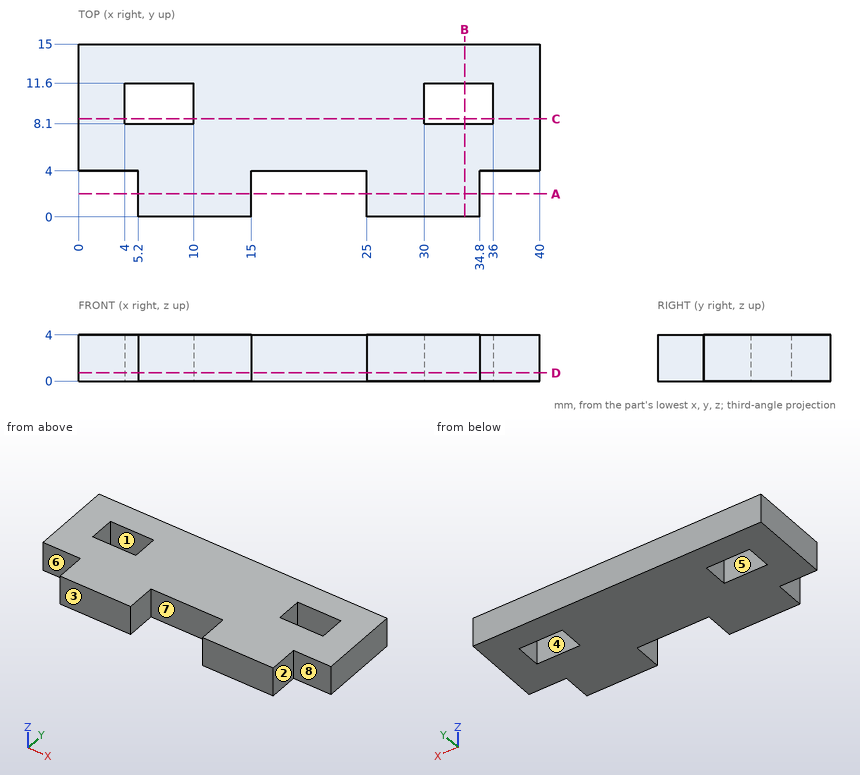
Geometry check sheet. Reference: drawing and pictorial views, mm from the part's lowest x, y, z. A direction names the side the tool comes from. Round coordinates to 2 decimals unless told otherwise and drop trailing zeros. Loops run counter-clockwise (first coordinate to the right, second up) from the corner with the lowest first, then second, coordinate; pieces in that order, holes last.
1. Sectioned sample at A-A on y = 2. Record the boundary of the cut face in (x, z).
2. Set-up check for the marked faces 5, 6, 7 and 8: record each of +Z, -Z, +X, -X, +Y, -Y from which the full face is reachable in a straight line by a thin tool's end or side.
3. Scan lines: probe 1 along X at (y, z) = (10.5, 0.2); probe 2 along Y at (x, z) = (5.5, 3.35); probe 3 along Y at (x, z) = (4.5, 3.65). Record each from-to range of solid material in increasing order.
4. Sectioned sample at C-C on y = 8.5. Record the boundary of the cut face in (x, z).
5. Sectioned sample at D-D on z = 0.7. Record the boundary of the cut face in (x, y), and give its area (3 significant figures).
6. Mould release check, pull along X, two halves, no side actions. Record for the marked faces 1, 2, 3 and 4: released by +X, released by -X, zero draft, split by the parting line, or undercut.
7. Gauge pin test, flat ends, axial feed: pin 1 Ø2 at (y, z) = (2, 1.5) entering from -X; pin 2 Ø2 at (y, z) = (2.5, 2.5) entering from +X; pin 3 Ø2 at (x, z) = (1.5, 2) entering from -Y. Record the tip position at first contact, or that the pin passes through.
8. Sectioned sample at B-B on x = 33.5. Record the boundary of the cut face in (y, z), and give its area (3 significant figures).
Recorded:
1. outline: (5.2, 0) - (15, 0) - (15, 4) - (5.2, 4) - close; (25, 0) - (34.8, 0) - (34.8, 4) - (25, 4) - close
2. face 5: +Z, -Z
2. face 6: +Z, -Z, -X, -Y
2. face 7: +Z, -Z, -Y
2. face 8: +Z, -Z, +X, -Y
3. probe 1: x = 0 to 4, 10 to 30, 36 to 40
3. probe 2: y = 0 to 8.1, 11.6 to 15
3. probe 3: y = 4 to 8.1, 11.6 to 15
4. outline: (0, 0) - (4, 0) - (4, 4) - (0, 4) - close; (10, 0) - (30, 0) - (30, 4) - (10, 4) - close; (36, 0) - (40, 0) - (40, 4) - (36, 4) - close
5. outline: (0, 4) - (5.2, 4) - (5.2, 0) - (15, 0) - (15, 4) - (25, 4) - (25, 0) - (34.8, 0) - (34.8, 4) - (40, 4) - (40, 15) - (0, 15) - close; hole (4, 8.1) - (10, 8.1) - (10, 11.6) - (4, 11.6) - close; hole (30, 8.1) - (36, 8.1) - (36, 11.6) - (30, 11.6) - close
5. area: 476 mm2
6. face 1: undercut
6. face 2: released by +X
6. face 3: zero draft
6. face 4: undercut
7. pin 1: stops at x = 5.2
7. pin 2: stops at x = 34.8
7. pin 3: stops at y = 4
8. outline: (0, 0) - (8.1, 0) - (8.1, 4) - (0, 4) - close; (11.6, 0) - (15, 0) - (15, 4) - (11.6, 4) - close
8. area: 46.0 mm2
